Input: dimensioned drawing with shaded views. Units: mm. Origin: part minimum x, y, z. A direction names the side the tool comes from. Round coordinates to 2 decimals unless told otherwise and drop trailing zeros. Loops run counter-clockwise (first coordinate to the right, second up) from the corner with the lowest first, then second, coordinate; pieces in that order, holes last. Notation, with made-up numbers: (-11.75, -16) - (1.25, -16) arc R25 ccw to (1.25, -3) - close; hole circle Ø5 at (66, 8.25). An arc over 180 degrees is marked (long way). Answer as a JSON object with one key per item and string values. Group by question number.
Item 1: Section C-C (x = 175.5). Return the cut outline in (y, z), plus the area to 3 significant figures.
Item 2: Section B-B (y = 43). Return the cut outline in (x, z).
Item 3: Reachability of the marked faces 1 and 2 from +Z, -Z, +X, -X, +Y, -Y: full face, straight path, thin tool, end or side. Return the list, or none.
Item 4: Line query: line 1 (Z direction, x = 10, y = 12.25); line 2 (X direction, y = 7.25, z = 94.5); line 3 (Y direction, x = 190, z = 19.5). Output: solid intervals per line, ascending.
Item 5: Section A-A (z = 74). Return the cut outline in (x, y).
Item 6: First-contact query: pin 1 (16.5 mm diameter, centred on x = 4, z = 56.5, fed in from +Y); pin 2 (9 mm diameter, centred on y = 28.5, z = 54.5, fed in from +X); pin 3 (9 mm diameter, centred on y = 38, z = 59, fed in from -X). Flat tips, straight axial feed; report the tip coordinate or a pass-through.
Item 7: Draft query along Y for the marked faces 3, 4 and 5. Return one class per face: released by +Y, released by -Y, zero draft, split by the parting line, or undercut.
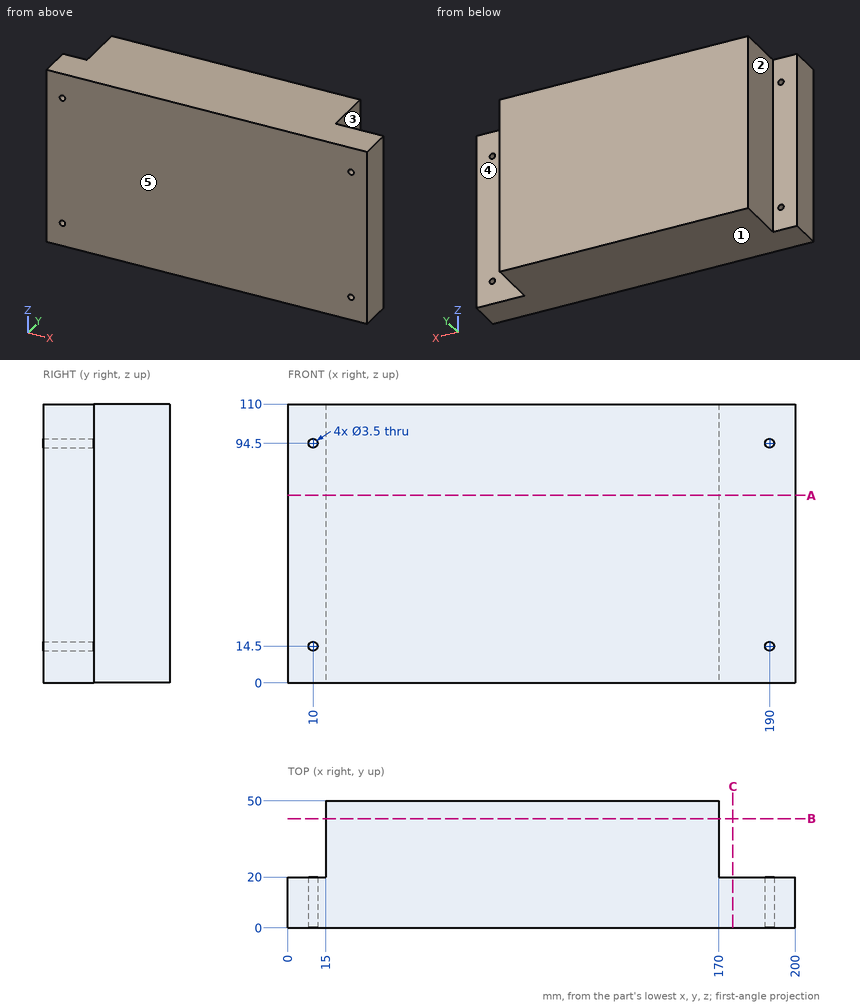
Values:
{
 "1": {"outline": "(0, 0) - (20, 0) - (20, 110) - (0, 110) - close", "area": "2,200 mm^2"},
 "2": {"outline": "(15, 0) - (170, 0) - (170, 110) - (15, 110) - close"},
 "3": {"face 1": "-Z, +X, -X, +Y, -Y", "face 2": "+Z, -Z, -X, +Y"},
 "4": {"line 1": "z = 0 to 12.75, 16.25 to 92.75, 96.25 to 110", "line 2": "x = 0 to 8.25, 11.75 to 188.25, 191.75 to 200", "line 3": "y = 0 to 20"},
 "5": {"outline": "(0, 0) - (200, 0) - (200, 20) - (170, 20) - (170, 50) - (15, 50) - (15, 20) - (0, 20) - close"},
 "6": {"pin 1": "stops at y = 20", "pin 2": "stops at x = 170", "pin 3": "stops at x = 15"},
 "7": {"face 3": "zero draft", "face 4": "released by +Y", "face 5": "released by -Y"}
}
